Geometry: final body of the model. Coordinates: model frame, mm. A direction names the side the tool comes from. Round coordinates to 2 decimals unless told otherwise and drop trailing zeros. Loops run counter-clockwise (first coordinate to the right, second up) from the corner with the lowest first, then second, coordinate; pieces in that order, holes last. Notation, with made-up numbers: M 16,51 L 60,51 A28 ccw 60,87 Z; hole C -21.75,59.5 d5. An arc over 180 degrees is marked long. Answer as a JSON object with one key per item and string values.
```python
from build123d import *

# Parameters (mm, degrees)
PAD020_DEPTH = 20
SKETCH023_R  = 2.2
PAD022_DEPTH = 10
SKETCH018_R  = 6
PAD016_DEPTH = 5
SKETCH020_R  = 4.5
PAD018_DEPTH = 12
SKETCH021_R  = 6.5
PAD019_DEPTH = 4.2
PAD021_DEPTH = 6


with BuildPart() as motor_linkage_hole_body001:
    # Sketch022 → Pad020 (new body)
    with BuildSketch(Plane.XY):
        with BuildLine():
            Line((-7, 2.236068), (-7, -2.236068))
            ThreePointArc((-7, -2.236068), (-5, -3), (-3, -2.236068))
            Line((-3, -2.236068), (-3, 2.236068))
            ThreePointArc((-3, 2.236068), (-5, 3), (-7, 2.236068))
        make_face()
    extrude(amount=-PAD020_DEPTH)


with BuildPart() as hole_fusion001:
    # Sketch023 → Pad022 (new body, symmetric)
    with BuildSketch(Plane.XY):
        with Locations((5.020646, 0)):
            Circle(SKETCH023_R)
    extrude(amount=PAD022_DEPTH, both=True)

    # Fusion012: union motor linkage hole body001
    add(motor_linkage_hole_body001.part)


with BuildPart() as motor_linkage_cut001:
    # Sketch018 → Pad016 (new body)
    with BuildSketch(Plane.XY):
        with Locations((5, 0)):
            Circle(SKETCH018_R)
    extrude(amount=PAD016_DEPTH)

    # Sketch020 → Pad018 (join)
    with BuildSketch(Plane.XY):
        with Locations((-5, 0)):
            Circle(SKETCH020_R)
    extrude(amount=-PAD018_DEPTH)

    # Sketch021 → Pad019 (join)
    with BuildSketch(Plane.XY):
        with Locations((-5, 0)):
            Circle(SKETCH021_R)
    extrude(amount=-PAD019_DEPTH)

    # Sketch017 → Pad021 (join)
    with BuildSketch(Plane.XY):
        with BuildLine():
            Line((-5, 8), (5, 8))
            ThreePointArc((5, -8), (13, 0), (5, 8))
            Line((-5, -8), (5, -8))
            ThreePointArc((-5, 8), (-13, 0), (-5, -8))
        make_face()
    extrude(amount=PAD021_DEPTH)

    # Cut006: cut hole fusion001
    add(hole_fusion001.part, mode=Mode.SUBTRACT)


solid = motor_linkage_cut001.part
```
1) Cut plane A-A on z = -3.25. Return the cut outline in (x, y).
Geometry results:
{"outline": "C -5,0 d13; hole M -7,-2.24 A3 ccw -3,-2.24 L -3,2.24 A3 ccw -7,2.24 Z"}
2) Cut plane D-D on y = -1.75. Return the cut outline in (x, z).
Geometry results:
{"outline": "M -12.81,0 L -11.26,0 L -11.26,-4.2 L -9.15,-4.2 L -9.15,-12 L -7,-12 L -7,0 L -3,0 L -3,-12 L -0.85,-12 L -0.85,-4.2 L 1.26,-4.2 L 1.26,0 L 3.69,0 L 3.69,6 L -12.81,6 Z; M 6.35,0 L 12.81,0 L 12.81,6 L 6.35,6 Z"}
3) Line query: probe 1 along Z at (x, y) = (0.5, 4.25); probe 2 along Y at (x, z) = (6.5, 3.5); probe 3 along Y at (x, z) = (4.5, 0.5). Output: solid intervals per line, ascending.
Geometry results:
{"probe 1": "0 to 6", "probe 2": "-7.86 to -1.63, 1.63 to 7.86", "probe 3": "-8 to -2.14, 2.14 to 8"}
4) Cut plane B-B on y = 0. Return the cut outline in (x, z).
Geometry results:
{"outline": "M -13,0 L -11.5,0 L -11.5,-4.2 L -9.5,-4.2 L -9.5,-12 L -7,-12 L -7,0 L -3,0 L -3,-12 L -0.5,-12 L -0.5,-4.2 L 1.5,-4.2 L 1.5,0 L 2.82,0 L 2.82,6 L -13,6 Z; M 7.22,0 L 13,0 L 13,6 L 7.22,6 Z"}
5) Cut plane C-C on z = 1. Return the cut outline in (x, y).
Geometry results:
{"outline": "M -5,-8 L 5,-8 A8 ccw 5,8 L -5,8 A8 ccw Z; hole C 5.02,0 d4.4"}
6) Pull-direction query (X, two-part tool) for faces 1 (the face through (-13, 0, 3)), 2 (the face through (-5, -3, -6)), 3 (the face through (3, -2, 0)), 4 (the face through (-3, 0, -6)); classes: +X half, -X half, draft (parallel to the pull), parting line (faces both ways), or undercut.
Geometry results:
{"face 1": "-X half", "face 2": "undercut", "face 3": "draft", "face 4": "undercut"}
7) First-contact query: pin 1 (1.2 mm diameter, centred on x = -4.5, y = -1.5, fed in from -Z); pin 2 (3 mm diameter, centred on y = -1, z = -5.5, fed in from -X); pin 3 (4 mm diameter, centred on x = 5.02, y = 0, fed in from +Z); pin 4 (3.5 mm diameter, centred on y = 0.5, z = -9, fed in from -X). Flat tips, straight axial feed; report the tip coordinate or a pass-through.
Geometry results:
{"pin 1": "z = 0", "pin 2": "x = -11.5", "pin 3": "through", "pin 4": "x = -9.5"}
8) Set-up query: faces 5 (the face through (0, 0, 6)), 6 (the face through (-5.59, 4.46, -8.05)). Return all of +Z, -Z, +X, -X, +Y, -Y with unobstructed straight access to the full face (end or side cutting, diameter ignored); none if empty.
Geometry results:
{"face 5": "+Z, +X, -X, +Y, -Y", "face 6": "-Z"}
